```python
from build123d import *

# Parameters (mm, degrees)
F1_DEPTH = 38.1
F2_R     = 5.08


with BuildPart() as f1:
    # F0 (on Top) → F1 (new body, symmetric)
    with BuildSketch(Plane.XY):
        with BuildLine():
            ThreePointArc((81.030455, -15.766034), (0, -82.55), (-81.030455, -15.766034))
            Line((-81.030455, -15.766034), (-84.908667, -15.766034))
            ThreePointArc((-84.908667, -15.766034), (-57.430588, -64.496335), (-5.852405, -86.16147))
            Line((-5.852405, -86.16147), (-5.852405, -98.86147))
            Line((-5.852405, -98.86147), (-3.312405, -98.86147))
            Line((-3.312405, -98.86147), (-4.620644, -93.952814))
            Line((-4.620644, -93.952814), (5.539356, -93.952814))
            Line((5.539356, -93.952814), (4.046382, -98.808473))
            Line((4.046382, -98.808473), (6.586382, -98.808473))
            Line((6.586382, -98.808473), (6.586382, -86.108473))
            ThreePointArc((6.586382, -86.108473), (57.704858, -64.251062), (84.908667, -15.766034))
            Line((84.908667, -15.766034), (81.030455, -15.766034))
        make_face()
    extrude(amount=F1_DEPTH, both=True)

    # F2
    f2_edges = [f1.edges().sort_by_distance(p)[0] for p in [
        (6.586382, -86.108473, 0),
        (-5.852405, -86.16147, 0),
    ]]
    fillet(f2_edges, radius=F2_R)


solid = f1.part
```
Part model, mm, in its own coordinate system. A direction names the side the tool comes from. Round coordinates to 2 decimals unless told otherwise and drop trailing zeros. Order: outer loops, then holes, each group sorted by start corner. A loop starts at its lowest first (then second) coordinate and runs counter-clockwise, first axis right, second up. Notation, with made-up numbers: M 23,11 L 58,11 A28 ccw 58,31 Z; hole C 83.25,19 d6. An arc over 180 degrees is marked long. Answer in a Markdown table with one row per item. Add a question column.
Q1. Cut at B-B on z = -32. Give the cut face in (x, y).
Q2. Cut at D-D on x = -56. Give the cut face in (y, z), and give its area (3 significant figures).
Q3. Wall check: L1, parallel to Y at x = -2.5, z = 22; L2, parallel to X at y = -33, z = -4; L3, parallel to X at y = -50, z = 33. Give the ranges that are in metal, low to high. Write a range as from..to.
Q4. Pin check, flat tips, straight feed: pin 1 (1.3 mm diameter, centred on x = 5.5, z = -7, fed in from -Y); pin 2 (3 mm diameter, centred on x = -55, z = -22.5, fed in from -Y); pin 3 (2 mm diameter, centred on x = 45, z = 6.5, fed in from +Y). Stop position of each tip, or through.
Q5. Cut at C-C on y = -30. Give the cut face in (x, z), and give its area (3 significant figures).
Q6. Mould opens along Y. For faces 1 (the face through (4.803, -96.347, 0.533)), 2 (the face through (83, -15.766, 1)), 3 (the face through (7.886, -87.299, -0.533)) say: +Y half, -Y half, draft (parallel to the pull), parting line (faces both ways), or undercut.
Q7. 3-axis set-ups, long thin cutter, end or side, ignore diameter. For faces 4 (the face through (-5.852, -95, 1)), 5 (the face through (0, -85, 38.1)), 6 (the face through (0, -93.953, 1)), 7 (the face through (1.593, -82.535, 0.533)), 8 (the face through (6.586, -95, 1)): which of +Z, -Z, +X, -X, +Y, -Y reach the whole face in a straight line?
Q8. Cut at A-A on y = -51.5. Give the cut face in (x, z).
Established:
| question | item | result |
|---|---|---|
| 1 | outline | M -84.91,-15.77 A86.36 ccw -10.33,-85.74 A5.08 cw -5.85,-90.78 L -5.85,-98.86 L -3.31,-98.86 L -4.62,-93.95 L 5.54,-93.95 L 4.05,-98.81 L 6.59,-98.81 L 6.59,-90.69 A5.08 cw 11.02,-85.65 A86.36 ccw 84.91,-15.77 L 81.03,-15.77 A82.55 cw -81.03,-15.77 Z |
| 2 | outline | M -65.74,-38.1 L -60.65,-38.1 L -60.65,38.1 L -65.74,38.1 Z |
| 2 | area | 388 mm2 |
| 3 | L1 | y = -93.95..-82.51 |
| 3 | L2 | x = -79.81..-75.67, 75.67..79.81 |
| 3 | L3 | x = -70.41..-65.68, 65.68..70.41 |
| 4 | pin 1 | stops at y = -98.81 |
| 4 | pin 2 | stops at y = -67.79 |
| 4 | pin 3 | stops at y = -68.55 |
| 5 | outline | M -80.98,-38.1 L -76.91,-38.1 L -76.91,38.1 L -80.98,38.1 Z; M 76.91,-38.1 L 80.98,-38.1 L 80.98,38.1 L 76.91,38.1 Z |
| 5 | area | 621 mm2 |
| 6 | face 1 | undercut |
| 6 | face 2 | +Y half |
| 6 | face 3 | -Y half |
| 7 | face 4 | +Z, -Z, -X, -Y |
| 7 | face 5 | +Z, +X, -X, +Y, -Y |
| 7 | face 6 | +Z, -Z |
| 7 | face 7 | +Z, -Z, +Y |
| 7 | face 8 | +Z, -Z, +X, -Y |
| 8 | outline | M -69.32,-38.1 L -64.52,-38.1 L -64.52,38.1 L -69.32,38.1 Z; M 64.52,-38.1 L 69.32,-38.1 L 69.32,38.1 L 64.52,38.1 Z |
